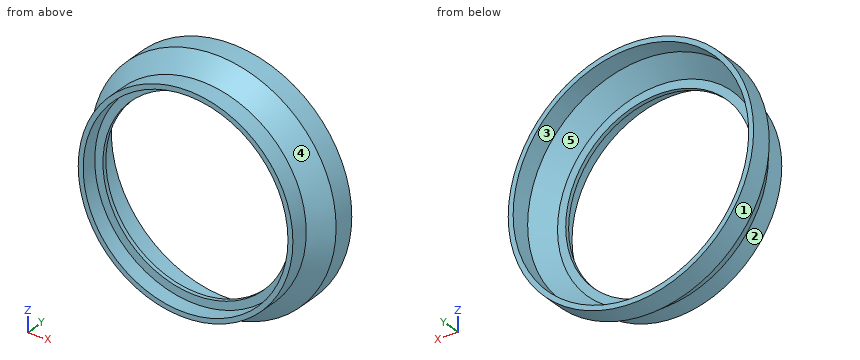
Autodesk Inventor part; units mm, degrees
ref_plane "YZ Plane" through (0, 0, 0) normal (1, 0, 0) x (0, 1, 0)
ref_plane "XZ Plane" through (0, 0, 0) normal (0, 1, 0) x (-1, 0, 0)
ref_plane "XY Plane" through (0, 0, 0) normal (0, 0, 1) x (1, 0, 0)
sketch "Esquisse2" plane through (0, 0, 0) normal (0, 0, 1) x (1, 0, 0)
  line L0 (-8.75, 36.8757) -> (-8.75, -38.6317)
  line L1 (20, 15) -> (20, 10)
  line L2 (16.25, 4) -> (16.25, 0)
  line L3 (20, 10) -> (16.25, 5)
  line L4 (16.25, 0) -> (17.45, 0)
  line L5 (17.45, 0) -> (17.45, 4.6)
  line L6 (17.45, 4.6) -> (21.2, 9.6)
  line L7 (21.2, 9.6) -> (21.2, 15)
  line L8 (21.2, 15) -> (20, 15)
  line L9 (16.25, 5) -> (14.25, 5)
  line L10 (14.25, 5) -> (14.25, 4)
  line L11 (14.25, 4) -> (16.25, 4)
  line L12 (-14.74, 0) -> (27.19, 0) construction
  line L13 (0, 51.9772) -> (0, -53.7332) construction
  point P0 (0, 0)
  dimension "d0" = 57.5
  dimension "d1" = 50
  dimension "d3" = 5
  dimension "d4" = 5
  dimension "d5" = 5
  dimension "d6" = 1.2
  dimension "d7" = 1.2
  dimension "d8" = 1.2
  dimension "d10" = 1
  dimension "d11" = 2
  dimension "d12" = 143.13
  dimension "d13" = 5
  dimension "d14" = 4.6
  dimension "d15" = 5.4
  dimension "d16" = 0
  dimension "d17" = 20
revolve "Révolution1" add sketch "Esquisse2" angle 360 about axis through (-8.75, 36.8757, 0) along (0, -1, 0)
properties part number "P012_Canon_AdaptCoudeTube"
Check sheet for the modelled part. Datum: model origin and axes. Units: mm. Face numbers are marked on the shaded views. A direction names the side the tool comes from. Round coordinates to 2 decimals unless told otherwise and drop trailing zeros. Loops run counter-clockwise (first coordinate to the right, second up) from the corner with the lowest first, then second, coordinate; pieces in that order, holes last. Notation, with made-up numbers: (19, 72.25) - (51, 72.25) arc R13 ccw to (51, 94.25) - close; hole circle Ø4 at (47, 70.5). An arc over 180 degrees is marked (long way). Answer as a JSON object with one key per item and string values. Group by question number.
Q1. Scan lines: line 1 along Z through (x, y) = (-8.75, 2.3); line 2 along X through (y, z) = (12.75, 9) (3 decimals); line 3 along Z through (x, y) = (-8.75, 12.95). Record each from-to range of solid material in increasing order. Write a range as [from, to].
Q2. Sectioned sample at A-A, the plane x = -8.75. Enter the section's corners in (y, z).
Q3. Mould release check, pull along X, two halves, no side actions. Record for the marked faces 3, 4 and 5: released by +X, released by -X, zero draft, split by the parting line, or undercut.
Q4. Gauge pin test, flat ends, axial feed: P1, Ø1.5, axis at y = 10.5, z = -7, coming from the -X side; P2, Ø1.5, axis at x = -13.5, y = 2, coming from the -Z side; P3, Ø1.5, axis at y = 13, z = -5, coming from the -X side. Record the tip position at first contact, or that the pin passes through.
Q5. Sectioned sample at C-C, the plane y = 2.5. Enter the section's corners in (x, z), plus the area to 3 significant figures.
Q6. Sectioned sample at B-B, the plane z = 0. Enter the section's corners in (x, y).
Q7. Set-up check for the marked faces 1 and 2: record each of +Z, -Z, +X, -X, +Y, -Y from which the full face is reachable in a straight line by a thin tool's end or side.
Q8. Sectioned sample at D-D, the plane y = 10.75. Enter the section's corners in (x, z).
Solution:
{
 "1": {"line 1": "z = [-26.2, -25], [25, 26.2]", "line 2": "x = [-37.316, -36.055], [18.555, 19.816]", "line 3": "z = [-29.95, -28.75], [28.75, 29.95]"},
 "2": {"outline": "(0, -26.2) - (4.6, -26.2) - (9.6, -29.95) - (15, -29.95) - (15, -28.75) - (10, -28.75) - (5, -25) - (5, -23) - (4, -23) - (4, -25) - (0, -25) - close; (0, 25) - (4, 25) - (4, 23) - (5, 23) - (5, 25) - (10, 28.75) - (15, 28.75) - (15, 29.95) - (9.6, 29.95) - (4.6, 26.2) - (0, 26.2) - close"},
 "3": {"face 3": "undercut", "face 4": "split by the parting line", "face 5": "undercut"},
 "4": {"P1": "stops at x = -38.04", "P2": "stops at z = -25.89", "P3": "stops at x = -38.4"},
 "5": {"outline": "circle Ø52.4 at (-8.75, 0); hole circle Ø50 at (-8.75, 0)", "area": "193 mm²"},
 "6": {"outline": "(-38.7, 9.6) - (-34.95, 4.6) - (-34.95, 0) - (-33.75, 0) - (-33.75, 4) - (-31.75, 4) - (-31.75, 5) - (-33.75, 5) - (-37.5, 10) - (-37.5, 15) - (-38.7, 15) - close; (14.25, 4) - (16.25, 4) - (16.25, 0) - (17.45, 0) - (17.45, 4.6) - (21.2, 9.6) - (21.2, 15) - (20, 15) - (20, 10) - (16.25, 5) - (14.25, 5) - close"},
 "7": {"face 1": "+Y, -Y", "face 2": "-Y"},
 "8": {"outline": "circle Ø59.9 at (-8.75, 0); hole circle Ø57.5 at (-8.75, 0)"}
}
